```python
from build123d import *

# Parameters (mm, degrees)
SKETCH1_R           = 13
SKETCH1_R_2         = 11
BOSS_EXTRUDE1_DEPTH = 3.5
SKETCH2_R           = 2.5
CUT_EXTRUDE3_DEPTH  = 1
CIRPATTERN1_COUNT   = 10


with BuildPart() as part:
    # Sketch1 → Boss-Extrude1 (new body, symmetric)
    with BuildSketch(Plane.XY):
        Circle(SKETCH1_R)
        Circle(SKETCH1_R_2, mode=Mode.SUBTRACT)
    extrude(amount=BOSS_EXTRUDE1_DEPTH, both=True)

    # Sketch2 → Cut-Extrude3 (cut)
    with BuildSketch(Plane(origin=(0, 13, 0), x_dir=(1, 0, 0), z_dir=(0, 1, 0))):
        Circle(SKETCH2_R)
    cut_extrude3 = extrude(amount=-CUT_EXTRUDE3_DEPTH, mode=Mode.SUBTRACT)

    # CirPattern1: Cut-Extrude3 ×10 about axis
    cirpattern1_axis = Axis((0, 0, 0), (0, 0, 1))
    for i in range(1, CIRPATTERN1_COUNT):
        add(cut_extrude3.rotate(cirpattern1_axis, i * 360 / CIRPATTERN1_COUNT), mode=Mode.SUBTRACT)


solid = part.part
```
Work out the finished part from the listing and answer in its coordinate system (mm). A direction names the side the tool comes from. Give positions to 0.01 mm unless a question says otherwise; leave off trailing zeros. Loops run counter-clockwise (first coordinate to the right, second up) from the corner with the lowest first, then second, coordinate; pieces in that order, holes last. Notation, with made-up numbers: (47.25, 49) -> (65.25, 49) arc R14 ccw to (65.25, 67) -> close; hole circle Ø11 at (44, 7). An arc over 180 degrees is marked (long way). Put each result on its own line as item: value. Start each with the question number.
Item 1: Which of the six approach directions +Z, -Z, +X, -X, +Y, -Y give full straight-line access (tool end or side, diameter ignored) to faces 4 (the face through (2.5, -12.4, -0.1)), 5 (the face through (-2.5, 12.4, -0.1)), 6 (the face through (7.08, -9.69, -0.04)), 7 (the face through (-2.38, -10.74, -0.05))?
Item 2: The part is cut by section B-B (y = 0). Give the vertices of the cut face in (x, z).
Item 3: The mould has two halves that part along X. Classify faces 1 (the face through (-10.316, -7.91, 0.049)), 2 (the face through (-11, 3, -3.5)), 3 (the face through (12.561, -1.455, -0.11)): released by +X, released by -X, zero draft, split by the parting line, or undercut.
Item 4: The part is cut by section C-C (y = 7.75). Give the vertices of the cut face in (x, z).
Item 5: Each of these flat-tipped pins is pushed along its axis until it touches: P1, Ø1, axis at y = -6, z = -2, coming from the -X side; P2, Ø3, axis at x = 0, z = 0, coming from the +Y side; P3, Ø2, axis at x = 5, z = -1.5, coming from the +Y side. Where does it stop, or does it pass through?
Item 6: Find the intervals of material crossed by L1, parallel to Y at x = 0, z = -1.25; L2, parallel to Z at x = 0, y = -12.6; L3, parallel to Z at x = -11, y = -6, in increasing order. Write a range as [from, to].
Item 7: The part is cut by section A-A (x = 0). Give the vertices of the cut face in (y, z).
Answers below:
1. face 4: -Y
1. face 5: +Y
1. face 6: none
1. face 7: +Z, -Z
2. outline: (-13, -3.5) -> (-11, -3.5) -> (-11, 3.5) -> (-13, 3.5) -> close; (11, -3.5) -> (13, -3.5) -> (13, 3.5) -> (11, 3.5) -> close
3. face 1: split by the parting line
3. face 2: zero draft
3. face 3: undercut
4. outline: (-10.44, -3.5) -> (-7.81, -3.5) -> (-7.81, 3.5) -> (-10.44, 3.5) -> close; (7.81, -3.5) -> (10.44, -3.5) -> (10.44, 3.5) -> (7.81, 3.5) -> close
5. P1: x = -11.78
5. P2: y = 12
5. P3: y = 12.37
6. L1: [-12, -11], [11, 12]
6. L2: [-3.5, -2.5], [2.5, 3.5]
6. L3: [-3.5, -0.96], [0.96, 3.5]
7. outline: (-13, -3.5) -> (-11, -3.5) -> (-11, 3.5) -> (-13, 3.5) -> (-13, 2.5) -> (-12, 2.5) -> (-12, -2.5) -> (-13, -2.5) -> close; (11, -3.5) -> (13, -3.5) -> (13, -2.5) -> (12, -2.5) -> (12, 2.5) -> (13, 2.5) -> (13, 3.5) -> (11, 3.5) -> close
